For this review, take the finished solid that the model builds, in its own axes (mm). A direction names the side the tool comes from. Give positions to 0.01 mm unless a question says otherwise; leave off trailing zeros. Order: outer loops, then holes, each group sorted by start corner. A loop starts at its lowest first (then second) coordinate and runs counter-clockwise, first axis right, second up. Notation, with made-up numbers: (75, -32.5) -> (83, -32.5) arc R11 cw to (83, -26.5) -> close; hole circle Ø5 at (18, -3.75). An arc over 180 degrees is marked (long way). Return JSON: item names as keys, results as strings. Group by question number.
1) Add section C-C (z = 11). Give the boundary of the cut face in (x, y).
2) The part is to be moulded in two halves that separate along X. For faces 3 (the face through (33.95, 14.79, -61.22)), 4 (the face through (47.77, 17.68, 27.26)), 5 (the face through (-1, 0, -1)), say which applies: released by +X, released by -X, zero draft, split by the parting line, or undercut.
3) Add section A-A (y = 16). Give the boundary of the cut face in (x, z).
4) To check wall thickness, follow line 1 along Y through (x, z) = (43, 18.5); line 2 along Z through (x, y) = (10, 22.75); line 3 along X through (y, z) = (15, 37). State the ranges of each line that lie inside material, in increasing order.
5) Add section B-B (x = 58). Give the boundary of the cut face in (y, z), then the cut area to 3 significant figures.
6) For faces 1 (the face through (-47.77, 17.68, -27.26)), 2 (the face through (-48, 30, 30)), list the 3-axis set-ups (+Z, -Z, +X, -X, +Y, -Y) from which the entire face can be reached by the end or side of a thin tool; tool diameter is ignored.
7) Add section D-D (z = 69). Give the boundary of the cut face in (x, y) (3 decimals), then the cut area to 3 significant figures.
8) Insertion check: P1, Ø2, axis at x = -51.5, z = 52.5, coming from the -Y side; P2, Ø8, axis at y = 17.5, z = 30.5, coming from the +X side; P3, Ø1, axis at x = -12.5, y = 6.5, coming from the -Z side; P4, Ø10, axis at x = 24, z = -7.5, coming from the +Y side. Each pin has a flat end and moves straight along its axis. Give the tip position at first contact, or say it passes through.
from build123d import *

# Parameters (mm, degrees)
BOSS_EXTRUDE1_DEPTH = 30
CUT_EXTRUDE1_DEPTH  = 25


with BuildPart() as part:
    # Sketch2 → Boss-Extrude1 (new body)
    with BuildSketch(Plane(origin=(0, 0, 0), x_dir=(1, 0, 0), z_dir=(0, 1, 0))):
        Polygon((-71.004000985, 38.623376049), (-68.950825331, -42.179580599), (2.053175654, -80.802956648), (71.004000985, -38.623376049), (68.950825331, 42.179580599), (-2.053175654, 80.802956648), align=None)
    extrude(amount=BOSS_EXTRUDE1_DEPTH)

    # Sketch3 → Cut-Extrude1 (cut)
    with BuildSketch(Plane(origin=(0, 30, 0), x_dir=(1, 0, 0), z_dir=(0, 1, 0))):
        Polygon((-32.478654732, 54.575363674), (-63.502978728, -0.839658241), (-31.024323997, -55.415021915), (32.478654732, -54.575363674), (63.502978728, 0.839658241), (31.024323997, 55.415021915), align=None)
    extrude(amount=-CUT_EXTRUDE1_DEPTH, mode=Mode.SUBTRACT)


solid = part.part
Evaluation:
{
 "1": {"outline": "(-69.74, 0) -> (70.3, 0) -> (70.3, 30) -> (56.87, 30) -> (56.87, 5) -> (-57.46, 5) -> (-57.46, 30) -> (-69.74, 30) -> close"},
 "2": {"face 3": "released by +X", "face 4": "undercut", "face 5": "zero draft"},
 "3": {"outline": "(-71, -38.62) -> (-2.05, -80.8) -> (68.95, -42.18) -> (71, 38.62) -> (2.05, 80.8) -> (-68.95, 42.18) -> close; hole (-63.5, 0.84) -> (-32.48, -54.58) -> (31.02, -55.42) -> (63.5, -0.84) -> (32.48, 54.58) -> (-31.02, 55.42) -> close"},
 "4": {"line 1": "0 to 5", "line 2": "-74.25 to -55.14, 54.87 to 75.94", "line 3": "-69.08 to -41.98, 42.32 to 70.96"},
 "5": {"outline": "(0, -48.14) -> (30, -48.14) -> (30, -10.09) -> (5, -10.09) -> (5, 8.99) -> (30, 8.99) -> (30, 46.58) -> (0, 46.58) -> close", "area": "2,360 mm^2"},
 "6": {"face 1": "+Y", "face 2": "+Z, -Z, +X, -X, +Y"},
 "7": {"outline": "(-19.645, 0) -> (21.347, 0) -> (21.347, 30) -> (-19.645, 30) -> close", "area": "1,230 mm^2"},
 "8": {"P1": "y = 0", "P2": "x = 70.9", "P3": "z = -74.72", "P4": "y = 5"}
}
